```python
from build123d import *

# Parameters (mm, degrees)
SKETCH2_W                        = 25.4
SKETCH2_H                        = 50.8
BOSS_EXTRUDE2_DEPTH              = 28.575
SKETCH3_W                        = 14.2875
SKETCH3_H                        = 22.225
SKETCH3_W_2                      = 9.525
CUT_EXTRUDE1_DEPTH               = 26.4
F_10_0_1935_DIAMETER_HOLE1_D     = 4.9149
F_10_0_1935_DIAMETER_HOLE1_DEPTH = 6.35
F_10_0_1935_DIAMETER_HOLE1_TIP   = 1.476584928
SKETCH8_R                        = 3.175
CUT_EXTRUDE3_DEPTH               = 37.5125
FILLET1_R                        = 6.35
FILLET2_R                        = 2.54
CHAMFER1_SIZE                    = 0.508
BOSS_EXTRUDE3_DEPTH              = 3.302


with BuildPart() as part:
    # Sketch2 → Boss-Extrude2 (new body)
    with BuildSketch(Plane(origin=(0, 0, 0), x_dir=(1, 0, 0), z_dir=(0, 1, 0))):
        Rectangle(SKETCH2_W, SKETCH2_H)
    extrude(amount=BOSS_EXTRUDE2_DEPTH)

    # Sketch3 → Cut-Extrude1 (cut, through all)
    with BuildSketch(Plane(origin=(12.7, 0, 0), x_dir=(0, 0, -1), z_dir=(1, 0, 0))):
        with Locations((-18.25625, 17.4625)):
            Rectangle(SKETCH3_W, SKETCH3_H)
        with Locations((18.25625, 17.4625)):
            Rectangle(SKETCH3_W, SKETCH3_H)
        with Locations((0, 17.4625)):
            Rectangle(SKETCH3_W_2, SKETCH3_H)
    extrude(amount=-CUT_EXTRUDE1_DEPTH, mode=Mode.SUBTRACT)

    # #10 (0.1935) Diameter Hole1
    with Locations(Plane(origin=(0, 6.35, 0), x_dir=(1, 0, 0), z_dir=(0, 1, 0))):
        with Locations((0, -17.4625), (0, 17.4625)):
            Hole(F_10_0_1935_DIAMETER_HOLE1_D / 2, depth=F_10_0_1935_DIAMETER_HOLE1_DEPTH)
            with Locations((0, 0, -(F_10_0_1935_DIAMETER_HOLE1_DEPTH + F_10_0_1935_DIAMETER_HOLE1_TIP / 2))):  # 118° drill point
                Cone(0, F_10_0_1935_DIAMETER_HOLE1_D / 2, F_10_0_1935_DIAMETER_HOLE1_TIP, mode=Mode.SUBTRACT)

    # Sketch8 → Cut-Extrude3 (cut, through all)
    with BuildSketch(Plane(origin=(0, 0, -11.1125), x_dir=(-1, 0, 0), z_dir=(0, 0, -1))):
        with Locations((0, 22.225)):
            Circle(SKETCH8_R)
    extrude(amount=-CUT_EXTRUDE3_DEPTH, mode=Mode.SUBTRACT)

    # Fillet1
    fillet1_edges = [part.edges().sort_by_distance(p)[0] for p in [
        (12.7, 28.575, 7.9375),
        (-12.7, 28.575, -7.9375),
        (-12.7, 28.575, 7.9375),
        (12.7, 28.575, -7.9375),
    ]]
    fillet(fillet1_edges, radius=FILLET1_R)

    # Fillet2
    fillet2_edges = [part.edges().sort_by_distance(p)[0] for p in [
        (12.7, 3.175, 25.4),
        (-12.7, 3.175, 25.4),
        (-12.7, 3.175, -25.4),
        (12.7, 3.175, -25.4),
    ]]
    fillet(fillet2_edges, radius=FILLET2_R)

    # Chamfer1
    chamfer1_edges = [part.edges().sort_by_distance(p)[0] for p in [
        (2.45745, 6.35, -17.4625),
        (2.45745, 0, -17.4625),
        (2.45745, 6.35, 17.4625),
        (2.45745, 0, 17.4625),
    ]]
    chamfer(chamfer1_edges, length=CHAMFER1_SIZE)

    # Sketch10 → Boss-Extrude3 (add, symmetric)
    with BuildSketch(Plane(origin=(0, 0, -7.9375), x_dir=(-1, 0, 0), z_dir=(0, 0, -1))):
        with BuildLine():
            Line((0, 25.4), (0, 19.05))
            ThreePointArc((0, 19.05), (-3.175, 22.225), (0, 25.4))
        make_face()
    boss_extrude3 = extrude(amount=BOSS_EXTRUDE3_DEPTH, both=True)

    # Mirror1: Boss-Extrude3 across plane
    add(boss_extrude3.mirror(Plane.XY))


solid = part.part
```
Could you check a few things on this model? Use its own coordinates, in mm. A direction names the side the tool comes from. Round coordinates to 2 decimals unless told otherwise and drop trailing zeros. Loops run counter-clockwise (first coordinate to the right, second up) from the corner with the lowest first, then second, coordinate; pieces in that order, holes last.
Q1. Thinking about a two-plate mould opening in Y: for faces 1 (the flat face through (1, 22, 11.24)), 2 (the flat face through (0, 17, -4.762)), 3 (the flat face through (0, 0, 0)), 4 (the flat face through (0, 22, -8)), which applies, pulls with the +Y half, pulls with the -Y half, needs draft (parallel to the pull), parting line crosses it, or undercut?
Q2. Please list where these lines run through material, in increasing order: L1, parallel to Z at x = 0, y = 2.3; L2, parallel to Z at x = 7, y = 15.5; L3, parallel to Y at x = 6.75, z = -16.
Q3. On a 3-axis mill with a long thin cutter (end or side, diameter ignored), from which of +Z, -Z, +X, -X, +Y, -Y can I reach the whole of each face in a straight line? I mean faces 5 (the flat face through (1, 22, -11.24)), 6 (the flat face through (0, 17, 11.112)), 7 (the flat face through (1, 22, 4.636)), 8 (the flat face through (0, 17, 4.762)), 9 (the flat face through (0, 3, 25.4)). Say none if no direction works.
Q4. I want a section at A-A (y = 23). Write out the boundary of the cut face in (x, z).
Q5. I want a section at D-D (z = -1.5). Write out the boundary of the cut face in (x, y), and give its area (3 significant figures).
Q6. For P1, Ø1.5, axis at x = 0, y = 20.5, coming from the +Z side; P2, Ø6.5, axis at x = -2, y = 15.5, coming from the -Z side; P3, Ø7, axis at y = 24, z = 6.5, coming from the -X side; P4, Ø11, axis at x = 6, y = 15, coming from the +Z side, each with a flat end and sliding along its axis, tell me the tip position at first contact or that it passes through.
Q7. I want a section at C-C (y = 5.25). Write out the boundary of the cut face in (x, z), and give its area (3 significant figures).
Answer below:
1. face 1: needs draft
1. face 2: undercut
1. face 3: pulls with the -Y half
1. face 4: undercut
2. L1: z = -25.4 to -19.92, -15.01 to 15.01, 19.92 to 25.4
2. L2: z = -11.11 to -4.76, 4.76 to 11.11
2. L3: y = 0 to 6.35
3. face 5: -Z, +X, -X, +Y
3. face 6: +Z
3. face 7: +X, -X, +Y
3. face 8: none
3. face 9: +Z, +X, -X, +Y, -Y
4. outline: (-12.65, -11.11) - (-3.08, -11.11) - (-3.08, -4.76) - (-12.65, -4.76) - close; (-12.65, 4.76) - (-3.08, 4.76) - (-3.08, 11.11) - (-12.65, 11.11) - close; (0, -11.24) - (3.08, -11.24) - (3.08, -11.11) - (12.65, -11.11) - (12.65, -4.76) - (3.08, -4.76) - (3.08, -4.64) - (0, -4.64) - close; (0, 4.64) - (3.08, 4.64) - (3.08, 4.76) - (12.65, 4.76) - (12.65, 11.11) - (3.08, 11.11) - (3.08, 11.24) - (0, 11.24) - close
5. outline: (-12.7, 0) - (12.7, 0) - (12.7, 6.35) - (-12.7, 6.35) - close
5. area: 161 mm2
6. P1: stops at z = 11.24
6. P2: stops at z = -11.11
6. P3: stops at x = -12.7
6. P4: stops at z = 11.11
7. outline: (-12.7, -22.86) arc R2.54 ccw to (-10.16, -25.4) - (10.16, -25.4) arc R2.54 ccw to (12.7, -22.86) - (12.7, 22.86) arc R2.54 ccw to (10.16, 25.4) - (-10.16, 25.4) arc R2.54 ccw to (-12.7, 22.86) - close; hole circle Ø4.91 at (0, -17.46); hole circle Ø4.91 at (0, 17.46)
7. area: 1,250 mm2
